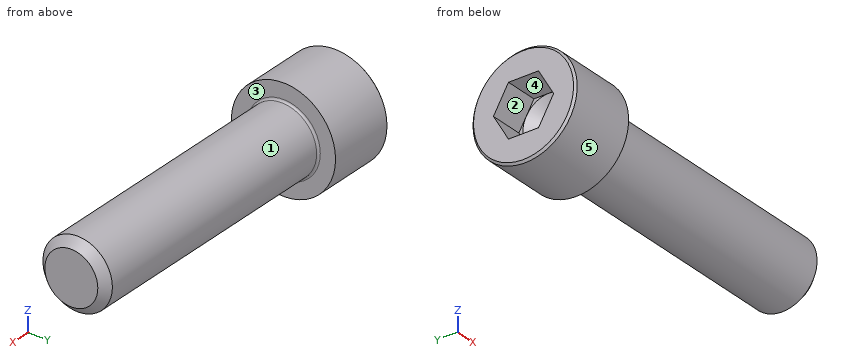
Autodesk Inventor part; units mm, degrees
ref_plane "screw_XY" through (0, 0, 0) normal (1, 0, 0) x (0, 0, -1)
ref_plane "screw_YZ" through (0, 0, 0) normal (0, 0, -1) x (0, 1, 0)
ref_plane "screw_ZX" through (0, 0, 0) normal (0, 1, 0) x (1, 0, 0)
sketch "Sketch_1" plane through (0, 0, 0) normal (0, 0, 1) x (1, 0, 0)
  line L0 (25.4, 0) -> (-6.35, 0)
  line L1 (-6.35, 0) -> (-6.35, 4.572)
  line L2 (-6.35, 4.572) -> (-6.1595, 4.7625)
  line L3 (-6.1595, 4.7625) -> (0, 4.7625)
  line L4 (0, 4.7625) -> (0, 3.3655)
  arc A0 (0, 3.3655) -> (0.1905, 3.175) centre (0.1905, 3.3655) ccw
  line L5 (0.1905, 3.175) -> (24.6443, 3.175)
  line L6 (24.6443, 3.175) -> (25.4, 2.4194)
  line L7 (25.4, 2.4194) -> (25.4, 0)
  line L8 (25.4, 0) -> (-6.35, 0)
revolve "Revolution1" add sketch "Sketch_1" angle 360 about axis through (25.4, 0, 0) along (1, 0, 0)
thread "Thread1"
sketch "Sketch_3" plane through (-6.35, 0, 0) normal (1, 0, 0) x (0, 0, -1)
  line L0 (-2.3813, -1.3748) -> (0, -2.7496)
  line L1 (0, -2.7496) -> (2.3813, -1.3748)
  line L2 (2.3813, -1.3748) -> (2.3813, 1.3748)
  line L3 (2.3813, 1.3748) -> (0, 2.7496)
  line L4 (0, 2.7496) -> (-2.3813, 1.3748)
  line L5 (-2.3813, 1.3748) -> (-2.3813, -1.3748)
extrude "Extrusion1" cut sketch "Sketch_3" along normal blind 3.048
sketch "Sketch_4" plane through (0, 0, 0) normal (0, 0, 1) x (1, 0, 0)
  line L0 (-1.9272, 0) -> (-3.302, 0)
  line L1 (-3.302, 0) -> (-3.302, 2.3813)
  line L2 (-3.302, 2.3813) -> (-1.9272, 0)
  line L3 (-1.9272, 0) -> (-3.302, 0)
revolve "Revolution2" cut sketch "Sketch_4" angle 360 about axis through (-1.9272, 0, 0) along (1, 0, 0)
ref_plane "screw_XY" through (0, 0, 0) normal (1, 0, 0) x (0, 0, -1)
ref_plane "screw_YZ" through (0, 0, 0) normal (0, 0, -1) x (0, 1, 0)
ref_plane "screw_ZX" through (0, 0, 0) normal (0, 1, 0) x (1, 0, 0)
ref_plane "screw1_XY" through (25.4, 0, 0) normal (1, 0, 0) x (0, 0, -1)
ref_plane "screw1_YZ" through (25.4, 0, 0) normal (0, 0, -1) x (0, 1, 0)
ref_plane "screw1_ZX" through (25.4, 0, 0) normal (0, 1, 0) x (1, 0, 0)
ref_plane "screw2_XY" through (20.32, 0, 0) normal (1, 0, 0) x (0, 0, -1)
ref_plane "screw2_YZ" through (20.32, 0, 0) normal (0, 0, -1) x (0, 1, 0)
ref_plane "screw2_ZX" through (20.32, 0, 0) normal (0, 1, 0) x (1, 0, 0)
ref_plane "to_tnut_XY" through (7.366, 0, 0) normal (1, 0, 0) x (0, 0, -1)
ref_plane "to_tnut_YZ" through (7.366, 0, 0) normal (0, 0, -1) x (0, 1, 0)
ref_plane "to_tnut_ZX" through (7.366, 0, 0) normal (0, 1, 0) x (1, 0, 0)
properties part number "3071"
Geometry: final body of the model. Coordinates: model frame, mm. Face numbers are marked on the shaded views. A direction names the side the tool comes from. Give positions to 0.01 mm unless a question says otherwise; leave off trailing zeros. Loops run counter-clockwise (first coordinate to the right, second up) from the corner with the lowest first, then second, coordinate; pieces in that order, holes last. Notation, with made-up numbers: (35, 55.25) - (54, 55.25) arc R27 ccw to (54, 75.25) - close; hole circle Ø4 at (-36, 42). An arc over 180 degrees is marked (long way). One line per question, with ' | ' between items. Start each with the question number.
(1) Reachability of the marked faces 4 and 5 from +Z, -Z, +X, -X, +Y, -Y: full face, straight path, thin tool, end or side. Return the list, or none.
(2) Pull-direction query (Z, two-part tool) for the marked faces 1, 2 and 3; classes: released by +Z, released by -Z, zero draft, split by the parting line, or undercut.
(3) Section query A-A on x = 14. Return loops of the section in (y, z) (3 decimals), then the cut area to 3 significant figures.
(4) Contact query for flat-ended pins moving along their axis: pin 1 (4 mm diameter, centred on x = 3.5, y = -0.5, fed in from +Z) (3 decimals); pin 2 (1 mm diameter, centred on x = 8, y = 0.5, fed in from -Z) (3 decimals); pin 3 (1.5 mm diameter, centred on x = -2.5, z = -2, fed in from -Y). Output: stop coordinate, or through.
(5) Ray query, line 1 (X direction, y = -3, z = -3.25); line 2 (Y direction, x = -4, z = 0.25); line 3 (Z direction, x = 17, y = 0) (3 decimals). Return the intervals inside material, ascending. Write a range as from..to.
The answers:
1) face 4: -X | face 5: +X, -X
2) face 1: split by the parting line | face 2: undercut | face 3: zero draft
3) outline: circle Ø6.35 at (0, 0) | area: 31.7 mm2
4) pin 1: z = 3.175 | pin 2: z = -3.175 | pin 3: y = -4.6
5) line 1: -6.35..0 | line 2: -4.76..-2.61, 2.61..4.76 | line 3: -3.175..3.175
